Read the model definition and answer for the solid it produces. Units are mm, in the model's axes. A direction names the side the tool comes from. Give positions to 0.01 mm unless a question says otherwise; leave off trailing zeros. Order: outer loops, then holes, each group sorted by start corner. A loop starts at its lowest first (then second) coordinate and runs counter-clockwise, first axis right, second up.
Item 1: A cutting plane is placed at B-B (z = 47). Write down the section's boundary in (x, y), plus the area to 3 significant figures.
Item 2: A cutting plane is placed at D-D (z = -35). Write down the section's boundary in (x, y).
Item 3: Which of the six approach directions +Z, -Z, +X, -X, +Y, -Y give full straight-line access (tool end or side, diameter ignored) to faces 4 (the face through (0, 66, 51.752)), 5 (the face through (-14.079, 12, 47)), 6 (the face through (-12, 12.1, -22.9))?
Item 4: A cutting plane is placed at A-A (x = 0). State how many separate pieces and enclosed holes the cut face has, plus the area to 3 significant figures.
Item 5: The mould has two halves that part along X. Classify faces 1 (the face through (14.079, 12, -13)), 2 (the face through (15.032, 3.531, -24.963)), 3 (the face through (0, 12, -5.955)): +X half, -X half, draft (parallel to the pull), parting line (faces both ways), or undercut.
Item 6: Find the intervals of material crossed by line 1 along Y through (x, z) = (4, -6.5); line 2 along Y through (x, z) = (-8.5, 63); line 3 along X through (y, z) = (13, -12), in increasing order.
Item 7: Given pin 1 Ø10.5 at (y, z) = (63.5, 41.5) entering from -X; pin 2 Ø3 at (y, z) = (17, -27) entering from -X; pin 3 Ø4 at (x, y) = (12.5, 53.5) entering from -Z; pin 4 Ø7.5 at (x, y) = (0, 31.05) entering from +Z, each flat-ended and moving along its own axis, determine where each tip first touches the part or whether it passes through.
Item 8: A cutting plane is placed at C-C (y = 58.5). Write down the section's boundary in (x, z) (3 decimals), plus the area to 3 significant figures.
from build123d import *

# Parameters (mm, degrees)
SKETCH1_R                      = 6.4135
BOSS_EXTRUDE1_DEPTH            = 34.29
CUT_EXTRUDE1_REACH             = 100.106
SKETCH3_W                      = 12.7
SKETCH3_H                      = 51.6425
CUT_EXTRUDE1_DIRECTION_2_REACH = 100.106
SKETCH5_R                      = 2.159
CUT_EXTRUDE2_DEPTH             = 86.858993575
SKETCH6_W                      = 25.4
SKETCH6_H                      = 8.47980016
BOSS_EXTRUDE2_DEPTH            = 17.4625
CUT_EXTRUDE9_START             = -6.35
SKETCH12_R                     = 14.478
CUT_EXTRUDE9_DEPTH             = 15.08125
FILLET4_R                      = 6.35
CHAMFER1_SIZE                  = 1.5875
CUT_EXTRUDE13_DEPTH            = 95.203417847
SKETCH16_W                     = 40.857524936
SKETCH16_H                     = 6.35
BOSS_EXTRUDE3_DEPTH            = 61.16
SKETCH17_R                     = 2.159
CUT_EXTRUDE14_DEPTH            = 6.35
FILLET5_R                      = 6.35
SKETCH18_W                     = 28.157524936
SKETCH18_H                     = 38.06
BOSS_EXTRUDE4_DEPTH            = 10.8
SKETCH19_R                     = 2.1
CUT_EXTRUDE15_DEPTH            = 40
SKETCH21_R                     = 3.5
CUT_EXTRUDE16_DEPTH            = 11
SKETCH22_R                     = 3.5
CUT_EXTRUDE17_DEPTH            = 11


with BuildPart() as part:
    # Sketch1 → Boss-Extrude1 (new body)
    # profile 1 of 3: a face of its own
    with BuildSketch(Plane.XY):
        with BuildLine():
            Line((12.7, 6.75), (20.428762468, 6.75))
            ThreePointArc((20.428762468, 6.75), (31.422640825, 35.602442589), (12.7, 60.154255663))
            Line((12.7, 60.154255663), (12.7, 6.75))
        make_face()
    # profile 2 of 3: a face of its own
    with BuildSketch(Plane.XY):
        Polygon((-47, 0.4), (-10.625, 0.4), (10.625, 0.4), (47, 0.4), (47, 6.75), (12.7, 6.75), (12.7, 69.8924), (-12.7, 69.8924), (-12.7, 6.75), (-47, 6.75), align=None)
        with Locations((0, 31.0549)):
            Circle(SKETCH1_R, mode=Mode.SUBTRACT)
    # profile 3 of 3: a face of its own
    with BuildSketch(Plane.XY):
        with BuildLine():
            ThreePointArc((-12.7, 60.154255663), (-31.422640825, 35.602442589), (-20.428762468, 6.75))
            Line((-20.428762468, 6.75), (-12.7, 6.75))
            Line((-12.7, 6.75), (-12.7, 60.154255663))
        make_face()
    extrude(amount=BOSS_EXTRUDE1_DEPTH)

    # Sketch3 → Cut-Extrude1 (cut, up to next)
    with BuildSketch(Plane(origin=(12.7, 0, 0), x_dir=(0, 0, -1), z_dir=(1, 0, 0)), mode=Mode.PRIVATE) as cut_extrude1_sk1:
        with Locations((-17.145, 44.07115)):
            Rectangle(SKETCH3_W, SKETCH3_H)
    cut_extrude1_tool1 = extrude(cut_extrude1_sk1.sketch, amount=-CUT_EXTRUDE1_REACH, mode=Mode.PRIVATE) & part.part
    add(cut_extrude1_tool1.solids().sort_by_distance((12.7, 44.07115, 17.145))[0], mode=Mode.SUBTRACT)

    # Sketch3 → Cut-Extrude1 direction 2 (cut, up to next)
    with BuildSketch(Plane(origin=(12.7, 0, 0), x_dir=(0, 0, -1), z_dir=(1, 0, 0)), mode=Mode.PRIVATE) as cut_extrude1_direction_2_sk1:
        with Locations((-17.145, 44.07115)):
            Rectangle(SKETCH3_W, SKETCH3_H)
    cut_extrude1_direction_2_tool1 = extrude(cut_extrude1_direction_2_sk1.sketch, amount=CUT_EXTRUDE1_DIRECTION_2_REACH, mode=Mode.PRIVATE) & part.part
    add(cut_extrude1_direction_2_tool1.solids().sort_by_distance((12.7, 44.07115, 17.145))[0], mode=Mode.SUBTRACT)

    # Sketch5 → Cut-Extrude2 (cut, through all)
    with BuildSketch(Plane(origin=(0, 6.75, 0), x_dir=(1, 0, 0), z_dir=(0, 1, 0))):
        with Locations(Location((40, -27.94, 0), (0, 0, 180))):
            Circle(SKETCH5_R)
        with Locations(Location((40, -6.35, 0), (0, 0, 180))):
            Circle(SKETCH5_R)
        with Locations(Location((-40, -6.35, 0), (0, 0, 180))):
            Circle(SKETCH5_R)
        with Locations(Location((-40, -27.94, 0), (0, 0, 180))):
            Circle(SKETCH5_R)
    extrude(amount=-CUT_EXTRUDE2_DEPTH, mode=Mode.SUBTRACT)

    # Sketch6 → Boss-Extrude2 (add)
    with BuildSketch(Plane.XY.offset(34.29)):
        with Locations((0, 65.65249992)):
            Rectangle(SKETCH6_W, SKETCH6_H)
    boss_extrude2 = extrude(amount=BOSS_EXTRUDE2_DEPTH)

    # Sketch12 → Cut-Extrude9 (cut)
    with BuildSketch(Plane.XY.offset(23.495).offset(CUT_EXTRUDE9_START)):
        with Locations((0, 31.0549)):
            Circle(SKETCH12_R)
    cut_extrude9 = extrude(amount=CUT_EXTRUDE9_DEPTH, mode=Mode.SUBTRACT)

    # Mirror4: Boss-Extrude2, Cut-Extrude9 across plane
    add(boss_extrude2.mirror(Plane(origin=(0, 0, 17.145), x_dir=(1, 0, 0), z_dir=(0, 0, -1))))
    add(cut_extrude9.mirror(Plane(origin=(0, 0, 17.145), x_dir=(1, 0, 0), z_dir=(0, 0, -1))), mode=Mode.SUBTRACT)

    # Fillet4
    fillet4_edges = [part.edges().sort_by_distance(p)[0] for p in [
        (47, 3.575, 0),
        (-47, 3.575, 0),
        (-47, 3.575, 34.29),
        (47, 3.575, 34.29),
    ]]
    fillet(fillet4_edges, radius=FILLET4_R)

    # Chamfer1
    chamfer1_edges = [part.edges().sort_by_distance(p)[0] for p in [
        (-7.476567629, 43.453021652, 10.795),
    ]]
    chamfer(chamfer1_edges, length=CHAMFER1_SIZE)

    # Sketch15 → Cut-Extrude13 (cut, through all)
    with BuildSketch(Plane(origin=(0, 6.75, 0), x_dir=(1, 0, 0), z_dir=(0, 1, 0))):
        with BuildLine():
            Line((20.428762468, 1.013392391), (20.428762468, -35.303392391))
            ThreePointArc((20.428762468, -35.303392391), (22.863261605, -34.54592678), (25.4, -34.29))
            Line((25.4, -34.29), (40.65, -34.29))
            ThreePointArc((40.65, -34.29), (45.140128061, -32.430128061), (47, -27.94))
            Line((47, -27.94), (47, -6.35))
            ThreePointArc((47, -6.35), (45.140128061, -1.859871939), (40.65, 0))
            Line((40.65, 0), (25.4, 0))
            ThreePointArc((25.4, 0), (22.863261605, 0.25592678), (20.428762468, 1.013392391))
        make_face()
        with BuildLine():
            Line((-40.65, 0), (-25.4, 0))
            ThreePointArc((-25.4, 0), (-22.863261605, 0.25592678), (-20.428762468, 1.013392391))
            Line((-20.428762468, 1.013392391), (-20.428762468, -35.303392391))
            ThreePointArc((-20.428762468, -35.303392391), (-22.863261605, -34.54592678), (-25.4, -34.29))
            Line((-25.4, -34.29), (-40.65, -34.29))
            ThreePointArc((-40.65, -34.29), (-45.140128061, -32.430128061), (-47, -27.94))
            Line((-47, -27.94), (-47, -6.35))
            ThreePointArc((-47, -6.35), (-45.140128061, -1.859871939), (-40.65, 0))
        make_face()
    extrude(amount=-CUT_EXTRUDE13_DEPTH, mode=Mode.SUBTRACT)

    # Sketch16 → Boss-Extrude3 (add, symmetric)
    with BuildSketch(Plane(origin=(0, 0, 17.145), x_dir=(-1, 0, 0), z_dir=(0, 0, -1))):
        with Locations((0, 3.575)):
            Rectangle(SKETCH16_W, SKETCH16_H)
    extrude(amount=BOSS_EXTRUDE3_DEPTH, both=True)

    # Sketch17 → Cut-Extrude14 (cut)
    with BuildSketch(Plane.XZ.offset(-0.4)):
        with Locations((15.5, 57.145)):
            Circle(SKETCH17_R)
        with Locations((-15.5, 57.145)):
            Circle(SKETCH17_R)
        with Locations((15.5, -22.855)):
            Circle(SKETCH17_R)
        with Locations((-15.5, -22.855)):
            Circle(SKETCH17_R)
    extrude(amount=-CUT_EXTRUDE14_DEPTH, mode=Mode.SUBTRACT)

    # Fillet5
    fillet5_edges = [part.edges().sort_by_distance(p)[0] for p in [
        (-20.428762468, 6.75, 17.145),
        (20.428762468, 6.75, 17.145),
        (-20.428762468, 3.575, -44.015),
        (20.428762468, 3.575, -44.015),
        (-20.428762468, 3.575, 78.305),
        (20.428762468, 3.575, 78.305),
    ]]
    fillet(fillet5_edges, radius=FILLET5_R)

    # Sketch18 → Boss-Extrude4 (add)
    with BuildSketch(Plane(origin=(0, 6.75, 0), x_dir=(1, 0, 0), z_dir=(0, 1, 0))):
        with Locations((0, -59.275)):
            Rectangle(SKETCH18_W, SKETCH18_H)
    boss_extrude4 = extrude(amount=BOSS_EXTRUDE4_DEPTH)

    # Mirror5: Boss-Extrude4 across plane
    add(boss_extrude4.mirror(Plane(origin=(0, 0, 17.145), x_dir=(1, 0, 0), z_dir=(0, 0, -1))))

    # Sketch19 → Cut-Extrude15 (cut)
    with BuildSketch(Plane(origin=(0, 0, -44.015), x_dir=(-1, 0, 0), z_dir=(0, 0, -1))):
        with Locations((8.5, 12.5549)):
            Circle(SKETCH19_R)
        with Locations((-8.5, 12.5549)):
            Circle(SKETCH19_R)
    cut_extrude15 = extrude(amount=-CUT_EXTRUDE15_DEPTH, mode=Mode.SUBTRACT)

    # Mirror6: Cut-Extrude15 across plane
    add(cut_extrude15.mirror(Plane(origin=(0, 0, 17.145), x_dir=(1, 0, 0), z_dir=(0, 0, -1))), mode=Mode.SUBTRACT)

    # Sketch21 → Cut-Extrude16 (cut)
    with BuildSketch(Plane(origin=(0, 6.75, 0), x_dir=(1, 0, 0), z_dir=(0, 1, 0))):
        with Locations((15.5, -57.145)):
            Circle(SKETCH21_R)
    cut_extrude16 = extrude(amount=CUT_EXTRUDE16_DEPTH, mode=Mode.SUBTRACT)

    # Sketch22 → Cut-Extrude17 (cut)
    with BuildSketch(Plane(origin=(0, 6.75, 0), x_dir=(1, 0, 0), z_dir=(0, 1, 0))):
        with Locations((-15.5, -57.145)):
            Circle(SKETCH22_R)
    cut_extrude17 = extrude(amount=CUT_EXTRUDE17_DEPTH, mode=Mode.SUBTRACT)

    # Mirror7: Cut-Extrude16, Cut-Extrude17 across plane
    add(cut_extrude16.mirror(Plane(origin=(0, 0, 17.145), x_dir=(1, 0, 0), z_dir=(0, 0, -1))), mode=Mode.SUBTRACT)
    add(cut_extrude17.mirror(Plane(origin=(0, 0, 17.145), x_dir=(1, 0, 0), z_dir=(0, 0, -1))), mode=Mode.SUBTRACT)


solid = part.part
Response values:
1. outline: (-20.43, 0.4) - (20.43, 0.4) - (20.43, 6.75) - (14.08, 6.75) - (14.08, 17.55) - (-14.08, 17.55) - (-14.08, 6.75) - (-20.43, 6.75) - close; (-12.7, 61.41) - (12.7, 61.41) - (12.7, 69.89) - (-12.7, 69.89) - close; hole circle Ø4.2 at (-8.5, 12.55); hole circle Ø4.2 at (8.5, 12.55)
1. area: 751 mm2
2. outline: (-20.43, 0.4) - (20.43, 0.4) - (20.43, 6.75) - (14.08, 6.75) - (14.08, 17.55) - (-14.08, 17.55) - (-14.08, 6.75) - (-20.43, 6.75) - close; hole circle Ø4.2 at (-8.5, 12.55); hole circle Ø4.2 at (8.5, 12.55)
3. face 4: +Z, +X, -X, +Y
3. face 5: +Z, -X, +Y
3. face 6: -X, +Y
4. separate pieces: 3
4. enclosed holes: 0
4. area: 2,820 mm2
5. face 1: +X half
5. face 2: undercut
5. face 3: draft
6. line 1: y = 0.4 to 17.55, 61.41 to 69.89
6. line 2: y = 0.4 to 10.45, 14.65 to 17.55
6. line 3: x = -14.08 to -10.55, -6.45 to 6.45, 10.55 to 14.08
7. pin 1: stops at x = -12.7
7. pin 2: stops at x = -14.08
7. pin 3: stops at z = 0
7. pin 4: passes through
8. outline: (-15.963, 0) - (15.963, 0) - (15.963, 10.795) - (-15.963, 10.795) - close; (-15.963, 23.495) - (15.963, 23.495) - (15.963, 34.29) - (-15.963, 34.29) - close
8. area: 689 mm2
